For this review, take the finished solid that the model builds, in its own axes (mm). Face numbers are marked on the shaded views. A direction names the side the tool comes from. Round coordinates to 2 decimals unless told otherwise and drop trailing zeros. Order: outer loops, then holes, each group sorted by start corner. A loop starts at its lowest first (then second) coordinate and runs counter-clockwise, first axis right, second up. Notation, with made-up numbers: M 35,36.5 L 59,36.5 A12 cw 59,46.5 Z; hole C -7.75,71 d4. An arc over 180 degrees is marked long. Use a Markdown table: item, result.
Autodesk Inventor part; units mm, degrees
ref_plane "Work Plane1" through (-8.5267, 21.9678, 110.0832) normal (0, 0, 1) x (1, 0, 0)
ref_plane "Work Plane3" through (-8.5267, -54.2322, 21.6832) normal (0, -1, 0) x (1, 0, 0)
ref_plane "YZ Plane" through (0, 0, 0) normal (1, 0, 0) x (0, 1, 0)
ref_plane "Work Plane1" through (-8.5267, 21.9678, 110.0832) normal (0, 0, 1) x (1, 0, 0)
sketch "Sketch1" plane through (-8.5267, 21.9678, 110.0832) normal (0, 0, 1) x (1, 0, 0)
  line L0 (3.95, 0) -> (3.95, -10.3)
  line L1 (3.95, 0) -> (3.95, -5.15)
  line L2 (4.8, 0) -> (4.8, -10.3)
  point P0 (8.5267, -21.9678)
ref_plane "Work Plane3" through (-8.5267, -54.2322, 21.6832) normal (0, -1, 0) x (1, 0, 0)
sketch "Sketch6" plane through (-8.5267, -54.2322, 21.6832) normal (0, -1, 0) x (1, 0, 0)
  line L0 (3.95, 0.85) -> (3.95, 11.35)
  line L1 (3.95, 12.3) -> (3.95, -0.1)
  line L2 (5.95, 4.6) -> (5.95, 7.6)
  line L3 (25.6, 12.1) -> (4.8, 12.1) construction
  line L4 (15.2, 12.1) -> (15.2, 0) construction
  line L5 (25.6, 0) -> (4.8, 0) construction
  line L6 (26.45, 12.3) -> (26.45, -0.1)
  line L7 (-0.85, 6.1) -> (31.25, 6.1) construction
  line L8 (31.25, 14.3) -> (-0.85, 14.3)
  line L9 (31.25, -2.1) -> (-0.85, -2.1)
  line L10 (-0.85, 14.3) -> (-0.85, -2.1)
  line L11 (31.25, 14.3) -> (31.25, -2.1)
  line L12 (3.95, 12.3) -> (26.45, 12.3)
  line L13 (3.95, -0.1) -> (26.45, -0.1)
  point P0 (5.95, 6.1)
  point P1 (3.95, 6.1)
  point P2 (-0.85, 6.1)
  point P3 (26.45, 6.1)
  point P4 (31.25, 6.1)
  dimension "d19" = 12.4
extrude "Extrusion4" add sketch "Sketch6" against normal blind 5
sketch "Sketch7" plane through (-8.5267, -54.2322, 21.6832) normal (0, -1, 0) x (1, 0, 0)
  line L0 (2.95, 4.6) -> (3.95, 4.6)
  line L1 (3.95, 4.6) -> (3.95, 7.6)
  line L2 (3.95, 7.6) -> (2.95, 7.6)
  line L3 (2.95, 7.6) -> (2.95, 4.6)
  line L4 (3.95, -0.1) -> (3.95, 12.3)
  line L5 (-0.85, 14.3) -> (-0.85, -2.1)
  point P0 (8.5267, -21.6832)
  point P1 (2.95, 6.1)
  point P2 (3.95, 6.1)
  dimension "d20" = 1
  dimension "d21" = 3
extrude "Extrusion5" cut sketch "Sketch7" against normal up to surface (5 mm away)
sketch "Sketch8" plane through (-8.5267, -54.2322, 21.6832) normal (0, -1, 0) x (1, 0, 0)
  line L0 (-0.85, 14.3) -> (-0.85, -2.1)
  line L1 (-0.85, 2.1) -> (-8.85, 2.1)
  line L2 (-8.85, 2.1) -> (-8.85, 10.1)
  line L3 (-8.85, 10.1) -> (-0.85, 10.1)
  line L4 (-0.85, 10.1) -> (-0.85, 2.1)
  line L5 (4.05, 11.35) -> (4.05, 0.85)
  circle A0 centre (-4.85, 6.1) radius 2
  point P0 (8.5267, -21.6832)
  point P1 (-8.85, 6.1)
  point P2 (4.05, 6.1)
  point P3 (-4.85, 2.1)
  dimension "d24" = 8
  dimension "d25" = 8
  dimension "d26" = 4
extrude "Extrusion6" add sketch "Sketch8" against normal up to surface (5 mm away)
ref_plane "Work Plane4" through (-4.5767, -54.2322, 27.7832) normal (0, 0, 1) x (1, 0, 0)
properties part number "SG90 360 Degree Servo Holder"
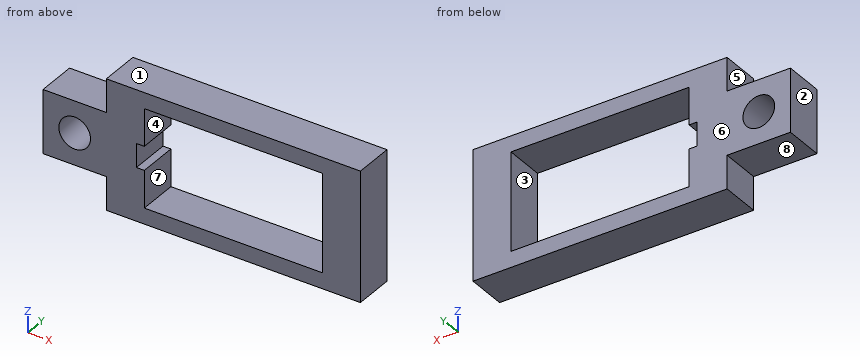
Q1. Draft analysis for pull direction X (two halves, no side actions). For the marked faces 1, 2, 3 and 4, state which applies: pulls with the +X half, pulls with the -X half, needs draft (parallel to the pull), parting line crosses it, or undercut.
Determined:
| item | result |
|---|---|
| face 1 | needs draft |
| face 2 | pulls with the -X half |
| face 3 | undercut |
| face 4 | undercut |
Q2. Clearance check with flat-ended pins moving along their axes: pin 1 (3.5 mm diameter, centred on x = -13.38, z = 27.78, fed in from -Y); pin 2 (2 mm diameter, centred on y = -52, z = 34.5, fed in from -X). State where each tip first meets the part, or that it passes through.
Determined:
| item | result |
|---|---|
| pin 1 | passes through |
| pin 2 | stops at x = -9.38 |
Q3. Add section D-D (z = 27.25). Write out the cut boundary in (x, y), then the cut area to 3 significant figures.
Determined:
| item | result |
|---|---|
| outline | M -17.38,-54.23 L -15.3,-54.23 L -15.3,-49.23 L -17.38,-49.23 Z; M -11.45,-54.23 L -5.58,-54.23 L -5.58,-49.23 L -11.45,-49.23 Z; M 17.92,-54.23 L 22.72,-54.23 L 22.72,-49.23 L 17.92,-49.23 Z |
| area | 63.7 mm^2 |
Q4. Wall thickness on line 1 along Z through (x, y) = (16, -53); line 2 along X through (y, z) = (-51.4, 25.25); line 3 along X through (y, z) = (-50, 33): over which ranges is each line inside the solid? List them lowest first. Write a range as [from, to].
Determined:
| item | result |
|---|---|
| line 1 | z = [19.58, 21.58], [33.98, 35.98] |
| line 2 | x = [-17.38, -4.58], [17.92, 22.72] |
| line 3 | x = [-9.38, -4.58], [17.92, 22.72] |
Q5. Add section B-B (x = 16). Write out the cut boundary in (y, z).
Determined:
| item | result |
|---|---|
| outline | M -54.23,19.58 L -49.23,19.58 L -49.23,21.58 L -54.23,21.58 Z; M -54.23,33.98 L -49.23,33.98 L -49.23,35.98 L -54.23,35.98 Z |
Q6. Add section A-A (z = 25). Write out the cut boundary in (x, y), then the cut area to 3 significant figures.
Determined:
| item | result |
|---|---|
| outline | M -17.38,-54.23 L -4.58,-54.23 L -4.58,-49.23 L -17.38,-49.23 Z; M 17.92,-54.23 L 22.72,-54.23 L 22.72,-49.23 L 17.92,-49.23 Z |
| area | 88.0 mm^2 |
Q7. Machinability: for the marked faces 5, 6, 7 and 8, which of the approach directions +Z, -Z, +X, -X, +Y, -Y give a long, thin tool a straight path to every point of the face, cutting with its end or side? Answer none if there is none.
Determined:
| item | result |
|---|---|
| face 5 | +Z, -X, +Y, -Y |
| face 6 | +Z, -Z, +X, -X, +Y |
| face 7 | +Y, -Y |
| face 8 | -Z, -X, +Y, -Y |
Q8. Add section C-C (y = -53.05). Write out the cut boundary in (x, z), then the cut area to 3 significant figures.
Determined:
| item | result |
|---|---|
| outline | M -17.38,23.78 L -9.38,23.78 L -9.38,19.58 L 22.72,19.58 L 22.72,35.98 L -9.38,35.98 L -9.38,31.78 L -17.38,31.78 Z; hole C -13.38,27.78 d4; hole M -5.58,26.28 L -4.58,26.28 L -4.58,21.58 L 17.92,21.58 L 17.92,33.98 L -4.58,33.98 L -4.58,29.28 L -5.58,29.28 Z |
| area | 296 mm^2 |
